Build history of the part. All positions in model axes, mm. Round coordinates to 2 decimals unless told otherwise and drop trailing zeros. Loops run counter-clockwise (first coordinate to the right, second up) from the corner with the lowest first, then second, coordinate; pieces in that order, holes last. Notation, with made-up numbers: M -12.5,-33 L 41.5,-33 A18 ccw 41.5,-1 Z; hole C 6,-32 d9. An arc over 180 degrees is marked long. One line per item, written item: value.
```python
from build123d import *

# Parameters (mm, degrees)
F1_DEPTH = 190.5
F2_R     = 6.35
F3_DEPTH = 21.9964
F6_D     = 6.35
F7_R     = 6.35
F8_DEPTH = 63.5


with BuildPart() as f1:
    # F0 (on Front) → F1 (new body)
    with BuildSketch(Plane.XZ):
        with BuildLine():
            Line((210.5406, 0), (12.1031, 0))
            ThreePointArc((12.1031, 0), (4.95935, -4.124446), (4.95935, 4.124446))
            Line((4.95935, 4.124446), (-24.4094, 54.992613))
            Line((-24.4094, 54.992613), (-35.4203, 48.649759))
            Line((-35.4203, 48.649759), (0, -12.7))
            Line((0, -12.7), (210.5406, -12.7))
            Line((210.5406, -12.7), (210.5406, 0))
        make_face()
    extrude(amount=F1_DEPTH)

    # F2 (on face) → F3 (join)
    with BuildSketch(Plane(origin=(5.50545, 0, 3.178573), x_dir=(0, 1, 0), z_dir=(0.866025, 0, 0.5))):
        with Locations((-25.554094, 34.4297)):
            Circle(F2_R)
    extrude(amount=F3_DEPTH)

    # F6 (through all)
    with Locations(Plane.XY):
        with Locations((108.9279, -12.7), (159.7279, -12.7), (108.9279, -76.2), (108.9279, -152.4)):
            Hole(F6_D / 2)

    # F7 (on face) → F8 (join)
    with BuildSketch(Plane.XY):
        with Locations((45.4533, -12.7)):
            Circle(F7_R)
    extrude(amount=F8_DEPTH)


solid = f1.part
```
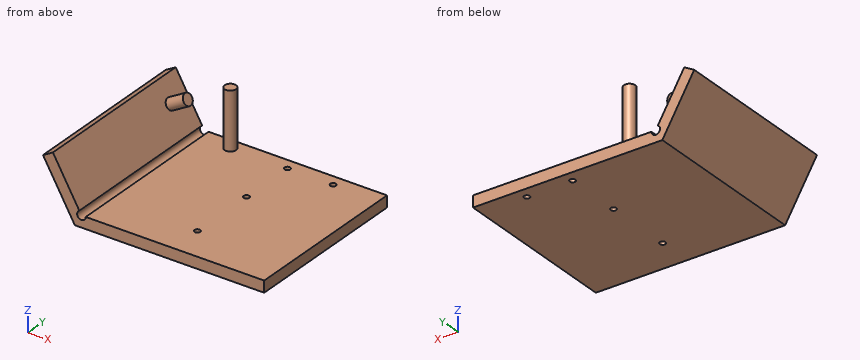
Item 1: Slice it at B-B, the plane y = -152.4. Give the cut face in (x, z) (1 decimal).
Check values:
outline: M -35.4,48.6 L 0,-12.7 L 105.8,-12.7 L 105.8,0 L 12.1,0 A4.8 cw long 5,4.1 L -24.4,55 Z; M 112.1,-12.7 L 210.5,-12.7 L 210.5,0 L 112.1,0 Z
Item 2: Slice it at C-C, the plane z = 14.5. Give the cut face in (x, y), and give its area (3 significant figures).
Check values:
outline: M -15.7,-190.5 L -1.03,-190.5 L -1.03,0 L -15.7,0 Z; C 45.45,-12.7 d12.7
area: 2,920 mm2
Item 3: Wall check: line 1 along Z through (x, y) = (142.5, -131.5); line 2 along X through (y, z) = (-171, 45.5); line 3 along Z through (x, y) = (-23, -120.5). Give the ranges that are in metal, low to high.
Check values:
line 1: z = -12.7 to 0
line 2: x = -33.6 to -18.93
line 3: z = 27.14 to 52.55
Item 4: Slice it at A-A, the plane y = -12.7. Give the cut face in (x, z) (1 decimal), and give its area (3 significant figures).
Check values:
outline: M -35.4,48.6 L 0,-12.7 L 105.8,-12.7 L 105.8,0 L 51.8,0 L 51.8,63.5 L 39.1,63.5 L 39.1,0 L 12.1,0 A4.8 cw long 5,4.1 L -24.4,55 Z; M 112.1,-12.7 L 156.6,-12.7 L 156.6,0 L 112.1,0 Z; M 162.9,-12.7 L 210.5,-12.7 L 210.5,0 L 162.9,0 Z
area: 4,080 mm2
Item 5: Slice it at D-D, the plane y = -122.5. Give the cut face in (x, z) (1 decimal).
Check values:
outline: M -35.4,48.6 L 0,-12.7 L 210.5,-12.7 L 210.5,0 L 12.1,0 A4.8 cw long 5,4.1 L -24.4,55 Z
Item 6: Drop flat-ended pins along their axis: P1, Ø10, axis at y = -35.5, z = -2.5, coming from the -X side; P2, Ø1.5, axis at y = -57, z = 41, coming from the -X side; P3, Ø8, axis at y = -144, z = 39.5, coming from the +X side; P4, Ø8.5, axis at x = 159.73, y = -12.7, coming from the -Z side. Give the stop position or say it passes through.
Check values:
P1: stops at x = -8.78
P2: stops at x = -31.44
P3: stops at x = -13.16
P4: stops at z = -12.7
